```python
from build123d import *

# Parameters (mm, degrees)
F0_W     = 75.82964
F0_H     = 7.62
F1_DEPTH = 38.1
F3_DEPTH = 3.81
F4_R     = 47.625
F5_DEPTH = 50.8
F6_R     = 31.75
F7_DEPTH = 50.801


with BuildPart() as f1:
    # F0 (on Front) → F1 (new body, symmetric)
    with BuildSketch(Plane.XZ):
        with Locations((-37.91482, 3.81)):
            Rectangle(F0_W, F0_H)
    extrude(amount=F1_DEPTH, both=True)

    # F2 (on Front) → F3 (join, symmetric)
    with BuildSketch(Plane.XZ):
        Polygon((-22.225, 50.8), (-64.990714, 7.62), (0, 7.62), (0, 50.8), align=None)
    extrude(amount=F3_DEPTH, both=True)

    # F4 (on face) → F5 (join)
    with BuildSketch(Plane.XY.offset(50.8)):
        with Locations((24.765, 0)):
            Circle(F4_R)
    extrude(amount=-F5_DEPTH)

    # F6 (on face) → F7 (cut, through all)
    with BuildSketch(Plane.XY.offset(50.8)):
        with Locations((24.765, 0)):
            Circle(F6_R)
    extrude(amount=-F7_DEPTH, mode=Mode.SUBTRACT)


solid = f1.part
```
Work out the finished part from the listing and answer in its coordinate system (mm). A direction names the side the tool comes from. Round coordinates to 2 decimals unless told otherwise and drop trailing zeros. Write each loop counter-clockwise with the first axis right and the second up, starting at its lowest first coordinate (ties: lowest second). Pieces come first, ordered by that corner, then holes. Notation, with made-up numbers: (-34.75, 32) -> (5.25, 32) arc R26 cw to (5.25, 51) -> close; hole circle Ø8 at (50, 30.5). An arc over 180 degrees is marked (long way). Write each question's results on one line, items separated by ' | '.
Q1. Section C-C, the plane y = 0 is taken. Write down the section's boundary in (x, z) (3 decimals).
Data:
outline: (-75.83, 0) -> (-6.985, 0) -> (-6.985, 50.8) -> (-22.86, 50.8) -> (-22.86, 50.159) -> (-64.991, 7.62) -> (-75.83, 7.62) -> close; (56.515, 0) -> (72.39, 0) -> (72.39, 50.8) -> (56.515, 50.8) -> close
Q2. Section D-D, the plane x = -32.5 is taken. Write down the section's boundary in (y, z), then the cut area to 3 significant figures.
Data:
outline: (-38.1, 0) -> (38.1, 0) -> (38.1, 7.62) -> (3.81, 7.62) -> (3.81, 40.43) -> (-3.81, 40.43) -> (-3.81, 7.62) -> (-38.1, 7.62) -> close | area: 831 mm^2
Q3. Flat-ended cylindrical pins translate along their axes: P1, Ø10, axis at x = -31, y = 2.5, coming from the -Z side; P2, Ø10, axis at x = -24, z = 10, coming from the -Y side; P3, Ø8, axis at y = 30.5, z = 39.5, coming from the -X side; P4, Ø4, axis at x = -56.5, z = 2.5, coming from the +Y side. Find the tip coordinate at first contact, or state that the pin passes through.
Data:
P1: z = 0 | P2: y = -38.1 | P3: x = -14.81 | P4: y = 38.1
Q4. Determine the mould class of faces 6 (the flat face through (-40, 38.1, 4)), 7 (the cylindrical face through (70.19, 14.31, 25.76)), 8 (the flat face through (-75.83, -1, 4)), 9 (the cylindrical face through (-6.954, 1.396, 25.756)) for opening direction X: released by +X, released by -X, zero draft, split by the parting line, or undercut.
Data:
face 6: zero draft | face 7: split by the parting line | face 8: released by -X | face 9: undercut
Q5. Section A-A, the plane z = 6 is taken. Write down the section's boundary in (x, y) (3 decimals).
Data:
outline: (-75.83, -38.1) -> (-3.81, -38.1) arc R47.625 ccw (long way) to (-3.81, 38.1) -> (-75.83, 38.1) -> close; hole circle Ø63.5 at (24.765, 0)
Q6. Straight lines are drawn through the part: line 1 along Z through (x, y) = (-64, 18); line 2 along X through (y, z) = (2, 8); line 3 along Y through (x, z) = (5.5, 48). For each, find the intervals that lie inside material, in ascending order. Write a range as [from, to].
Data:
line 1: [0, 7.62] | line 2: [-64.61, -6.92], [56.45, 72.35] | line 3: [-43.55, -25.24], [25.24, 43.55]
Q7. Which of the six approach directions +Z, -Z, +X, -X, +Y, -Y give full straight-line access (tool end or side, diameter ignored) to faces 1 (the flat face through (-35, 3.81, 20)), 2 (the flat face through (-40, -38.1, 4)), 3 (the flat face through (35, -31, 50.8)), 4 (the flat face through (-35, -3.81, 20)), 5 (the flat face through (-48, -9, 7.62))?
Data:
face 1: +Z, -X, +Y | face 2: +Z, -Z, -X, -Y | face 3: +Z, +X, -X, +Y, -Y | face 4: +Z, -X, -Y | face 5: +Z, -X
Q8. Section B-B, the plane x = 44 is taken. Write down the section's boundary in (y, z).
Data:
outline: (-43.57, 0) -> (-25.26, 0) -> (-25.26, 50.8) -> (-43.57, 50.8) -> close; (25.26, 0) -> (43.57, 0) -> (43.57, 50.8) -> (25.26, 50.8) -> close
